```python
from build123d import *

# Parameters (mm, degrees)
F1_DEPTH = 160
F2_W     = 10
F2_H     = 10
F3_DEPTH = 60
F5_DEPTH = 60


with BuildPart() as f1:
    # F0 (on Front) → F1 (new body, symmetric)
    with BuildSketch(Plane.XZ):
        Polygon((30, -15), (30, 15), (-8, 15), (-14.8404028665, -3.7938524157), (-22.8404028665, -3.7938524157), (-16, 15), (-30, 15), (-30, -15), (8, -15), (14.8404028665, 3.7938524157), (22.8404028665, 3.7938524157), (16, -15), align=None)
    extrude(amount=F1_DEPTH, both=True)

    # F2 (on face) → F3 (cut)
    with BuildSketch(Plane.XY.offset(15)):
        Rectangle(F2_W, F2_H)
    extrude(amount=-F3_DEPTH, mode=Mode.SUBTRACT)

    # F4 (on face) → F5 (cut)
    with BuildSketch(Plane.YZ.offset(30)):
        Polygon((0, 7.5), (0, 15), (-160, 15), (-160, -15), (0, -15), (0, -7.5), (-20, 0), align=None)
        Polygon((20, 15), (0, 15), (0, 7.5), align=None)
        Polygon((0, -15), (20, -15), (0, -7.5), align=None)
    extrude(amount=-F5_DEPTH, mode=Mode.SUBTRACT)


solid = f1.part
```
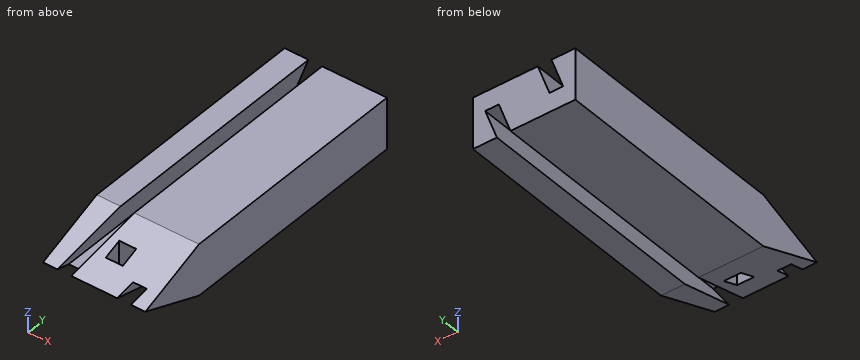
Build history of the part. All positions in model axes, mm. Round coordinates to 2 decimals unless told otherwise and drop trailing zeros. Write each loop counter-clockwise with the first axis right and the second up, starting at its lowest first coordinate (ties: lowest second). Pieces come first, ordered by that corner, then holes. Notation, with made-up numbers: (81, 62) - (107, 62) arc R35 cw to (107, 95) - close; hole circle Ø5 at (32.25, 82.5). An arc over 180 degrees is marked (long way). Write each question's results on one line, items separated by ' | '. Start each with the question number.
Item 1: Saw through at D-D (x = -11.5). Write the cut outline in (y, z).
Item 2: Saw through at C-C (x = 18). Write the cut outline in (y, z).
Item 3: Saw through at B-B (z = 11). Write the cut outline in (x, y), and give its area (3 significant figures).
Item 4: Drop a flat-ended pin along its axis: P1, Ø3, axis at x = -21.5, y = 2, coming from the -Z side. Give the stop position or say it passes through.
Item 5: Wall check: L1, parallel to X at y = 7.5, z = 2.5; L2, parallel to X at y = 90, z = -3.5; L3, parallel to X at y = 114, z = -6. Give the ranges that are in metal, low to high. Write a range as [from, to].
Item 6: Saw through at A-A (y = 88.5). Write the cut outline in (x, z), and give its area (3 significant figures).
Results are:
1) outline: (-20, 0) - (20, -15) - (160, -15) - (160, 5.38) - (-5.64, 5.38) - close
2) outline: (-9.88, 3.79) - (160, 3.79) - (160, 15) - (20, 15) - close; (5.35, -9.51) - (20, -15) - (160, -15) - (160, -9.51) - close
3) outline: (-30, 9.33) - (-17.46, 9.33) - (-17.46, 160) - (-30, 160) - close; (-9.46, 9.33) - (30, 9.33) - (30, 160) - (-9.46, 160) - close | area: 7,830 mm²
4) P1: stops at z = -8.81
5) L1: x = [-30, -20.55], [-12.55, 14.37], [22.37, 30] | L2: x = [-30, -22.73], [-14.73, 12.19], [20.19, 30] | L3: x = [-30, 11.28], [19.28, 30]
6) outline: (-30, -15) - (8, -15) - (14.84, 3.79) - (22.84, 3.79) - (16, -15) - (30, -15) - (30, 15) - (-8, 15) - (-14.84, -3.79) - (-22.84, -3.79) - (-16, 15) - (-30, 15) - close | area: 1,500 mm²
